from build123d import *

# Parameters (mm, degrees)
SKETCH1_W           = 60
SKETCH1_H           = 40
BOSS_EXTRUDE1_DEPTH = 20
SKETCH2_R           = 5
CUT_EXTRUDE1_DEPTH  = 42.231056256


with BuildPart() as part:
    # Sketch1 → Boss-Extrude1 (new body)
    with BuildSketch(Plane(origin=(0, 0, 0), x_dir=(1, 0, 0), z_dir=(0, 1, 0))):
        Rectangle(SKETCH1_W, SKETCH1_H)
    extrude(amount=BOSS_EXTRUDE1_DEPTH)

    # Sketch2 → Cut-Extrude1 (cut, through all)
    with BuildSketch(Plane(origin=(0, 20, 0), x_dir=(1, 0, 0), z_dir=(0, 1, 0))):
        with Locations(Location((20, 0, 0), (0, 0, 270))):
            Circle(SKETCH2_R)
    cut_extrude1 = extrude(amount=-CUT_EXTRUDE1_DEPTH, mode=Mode.SUBTRACT)

    # Mirror1: Cut-Extrude1 across plane
    add(cut_extrude1.mirror(Plane(origin=(0, 0, 0), x_dir=(0, 0, 1), z_dir=(1, 0, 0))), mode=Mode.SUBTRACT)


solid = part.part
The model under review builds one solid part; all positions refer to its coordinate system, in mm. Give positions to 0.01 mm unless a question says otherwise; leave off trailing zeros. Order: outer loops, then holes, each group sorted by start corner. A loop starts at its lowest first (then second) coordinate and runs counter-clockwise, first axis right, second up. Notation, with made-up numbers: M 87.5,6.5 L 144.5,6.5 A9 cw 144.5,14.5 Z; hole C 2,87.25 d10. An arc over 180 degrees is marked long. One line per question, with ' | ' between items. Start each with the question number.
1) Consider section A-A, the plane x = -20. Give the boundary of the cut face in (y, z).
2) Mouldability with a two-part tool opening along Z and no side actions: class faces 1 (the face through (-15.12, 10.14, -1.08)), 2 (the face through (15.12, 10.14, -1.08)), 3 (the face through (0, 20, 0)), 4 (the face through (0, 10, -20)) as pulls with the +Z half, pulls with the -Z half, needs draft (parallel to the pull), parting line crosses it, or undercut.
3) Consider section B-B, the plane z = 0. Give the boundary of the cut face in (x, y), then the cut area to 3 significant figures.
4) Clearance check with flat-ended pins moving along their axes: P1, Ø9, axis at x = 20, z = 0, coming from the -Y side; P2, Ø11.5, axis at x = -20, z = 0, coming from the +Y side. State where each tip first meets the part, or that it passes through.
5) Consider section C-C, the plane y = 18.5. Give the boundary of the cut face in (x, z).
6) Wall thickness on L1, parallel to X at y = 9.75, z = 0; L2, parallel to Z at x = -20, y = 9.5; L3, parallel to X at y = 18.5, z = 4: over which ranges is each line inside the solid? List them lowest first. Write a range as from..to.
Found:
1) outline: M 0,-20 L 20,-20 L 20,-5 L 0,-5 Z; M 0,5 L 20,5 L 20,20 L 0,20 Z
2) face 1: undercut | face 2: undercut | face 3: needs draft | face 4: pulls with the -Z half
3) outline: M -30,0 L -25,0 L -25,20 L -30,20 Z; M -15,0 L 15,0 L 15,20 L -15,20 Z; M 25,0 L 30,0 L 30,20 L 25,20 Z | area: 800 mm²
4) P1: passes through | P2: stops at y = 20
5) outline: M -30,-20 L 30,-20 L 30,20 L -30,20 Z; hole C -20,0 d10; hole C 20,0 d10
6) L1: x = -30..-25, -15..15, 25..30 | L2: z = -20..-5, 5..20 | L3: x = -30..-23, -17..17, 23..30
